```python
from build123d import *

# Parameters (mm, degrees)
F0_W     = 215
F0_H     = 215
F1_DEPTH = 15
F2_T     = -3.5
F3_R     = 11.5
F3_R_2   = 8.05
F4_DEPTH = 15
F5_R     = 5


with BuildPart() as f1:
    # F0 (on Top) → F1 (new body)
    with BuildSketch(Plane.XY):
        with Locations((107.5, 107.5)):
            Rectangle(F0_W, F0_H)
    extrude(amount=F1_DEPTH)

    # F2
    f2_openings = [f1.faces().sort_by_distance(p)[0] for p in [
        (107.5, 107.5, 15),
    ]]
    offset(amount=F2_T, openings=f2_openings)

    # F3 (on face) → F4 (join, through all)
    with BuildSketch(Plane(origin=(0, 0, 0), x_dir=(1, 0, 0), z_dir=(0, 0, -1))):
        with Locations((11.5, -11.5)):
            Circle(F3_R)
        with Locations((11.5, -11.5)):
            Circle(F3_R_2, mode=Mode.SUBTRACT)
        with Locations((11.5, -203.5)):
            Circle(F3_R)
        with Locations((11.5, -203.5)):
            Circle(F3_R_2, mode=Mode.SUBTRACT)
        with Locations((203.5, -11.5)):
            Circle(F3_R)
        with Locations((203.5, -11.5)):
            Circle(F3_R_2, mode=Mode.SUBTRACT)
        with Locations((203.5, -203.5)):
            Circle(F3_R)
        with Locations((203.5, -203.5)):
            Circle(F3_R_2, mode=Mode.SUBTRACT)
    extrude(amount=-F4_DEPTH)

    # F5
    f5_edges = [f1.edges().sort_by_distance(p)[0] for p in [
        (19.631728, 195.368272, 3.5),
        (107.5, 211.5, 3.5),
        (3.5, 107.5, 3.5),
        (195.368272, 195.368272, 3.5),
        (211.5, 107.5, 3.5),
        (19.631728, 19.631728, 3.5),
        (107.5, 3.5, 3.5),
        (195.368272, 19.631728, 3.5),
    ]]
    fillet(f5_edges, radius=F5_R)


solid = f1.part
```
The listing builds one solid part. Answer for the finished solid, in the listing's coordinates (mm). A direction names the side the tool comes from. Round coordinates to 2 decimals unless told otherwise and drop trailing zeros. Loops run counter-clockwise (first coordinate to the right, second up) from the corner with the lowest first, then second, coordinate; pieces in that order, holes last.
Q1. Which of the six approach directions +Z, -Z, +X, -X, +Y, -Y give full straight-line access (tool end or side, diameter ignored) to faces 3 (the face through (106, 0, 7)), 4 (the face through (5, 108.73, 4.93))?
Q2. Find the intervals of material crossed by line 1 (Y direction, x = 11.5, z = 8.75); line 2 (Y direction, x = 157, z = 13), in increasing order.
Q3. Section A-A, the plane z = 11.75 is taken. Determine the outline of the cut face in (x, y), then the cut area to 3 significant figures.
Q4. Section B-B, the plane x = 78 is taken. Determine the outline of the cut face in (y, z), then the cut area to 3 significant figures.
Q5. For a pull along X with two mould halves and no side action, classify faces 1 (the face through (67, 212, 15)), 2 (the face through (195.19, 19.45, 11.7)) as released by +X, released by -X, zero draft, split by the parting line, or undercut.
Q6. Given pin 1 Ø4 at (x, y) = (180.5, 54.5) entering from +Z; pin 2 Ø6 at (y, z) = (144, 6.5) entering from -X, each flat-ended and moving along its own axis, determine where each tip first touches the part or whether it passes through.
Completed:
1. face 3: +Z, -Z, +X, -X, -Y
1. face 4: +Z
2. line 1: y = 0 to 3.5, 19.55 to 23, 192 to 195.45, 211.5 to 215
2. line 2: y = 0 to 3.5, 211.5 to 215
3. outline: (0, 0) - (215, 0) - (215, 215) - (0, 215) - close; hole (3.5, 10.6) arc R8.05 ccw to (10.6, 3.5) - (12.4, 3.5) arc R8.05 ccw (long way) to (3.5, 12.4) - close; hole (3.5, 19.76) arc R11.5 cw to (19.76, 3.5) - (195.24, 3.5) arc R11.5 cw to (211.5, 19.76) - (211.5, 195.24) arc R11.5 cw to (195.24, 211.5) - (19.76, 211.5) arc R11.5 cw to (3.5, 195.24) - close; hole (3.5, 202.6) arc R8.05 ccw (long way) to (12.4, 211.5) - (10.6, 211.5) arc R8.05 ccw to (3.5, 204.4) - close; hole (202.6, 3.5) - (204.4, 3.5) arc R8.05 ccw to (211.5, 10.6) - (211.5, 12.4) arc R8.05 ccw (long way) to start; hole (202.6, 211.5) arc R8.05 ccw (long way) to (211.5, 202.6) - (211.5, 204.4) arc R8.05 ccw to (204.4, 211.5) - close
3. area: 3,490 mm2
4. outline: (0, 0) - (215, 0) - (215, 15) - (211.5, 15) - (211.5, 8.5) arc R5 cw to (206.5, 3.5) - (8.5, 3.5) arc R5 cw to (3.5, 8.5) - (3.5, 15) - (0, 15) - close
4. area: 844 mm2
5. face 1: zero draft
5. face 2: undercut
6. pin 1: stops at z = 3.5
6. pin 2: stops at x = 0
